Build history of the part. All positions in model axes, mm. Give positions to 0.01 mm unless a question says otherwise; leave off trailing zeros. Write each loop counter-clockwise with the first axis right and the second up, starting at its lowest first coordinate (ties: lowest second). Pieces come first, ordered by that corner, then holes. Notation, with made-up numbers: (0, 71.25) -> (43, 71.25) arc R18 cw to (43, 91.25) -> close; hole circle Ø8 at (-17.5, -27). An arc over 180 degrees is marked (long way). Put each result on its own line as item: value. Start each with the question number.
Item 1: Drill centre lines: line 1 along Y through (x, z) = (0.5, -5); line 2 along X through (y, z) = (18.5, -2.25); line 3 along Y through (x, z) = (0, -1.5). Where is each one in solid material? Low to high.
Item 2: Two-plate mould, pull along Y, no slides. Class faces 1 (the cylindrical face through (5.961, -26.846, -0.14)), 2 (the flat face through (-17, -22, -10)): pulls with the +Y half, pulls with the -Y half, needs draft (parallel to the pull), parting line crosses it, or undercut.
Item 3: Slice it at C-C, the plane z = -3. List the corners of the cut face in (x, y), plus the area to 3 significant figures.
Item 4: Slice it at A-A, the plane y = 0. List the corners of the cut face in (x, z), plus the area to 3 significant figures.
Item 5: Flat gauge pins, fed straight in: pin 1 Ø8 at (x, z) = (21.5, 4.5) entering from -Y; pin 2 Ø1.5 at (x, z) = (18, -8) entering from -Y; pin 3 Ø5 at (x, z) = (27, 3) entering from -Y; pin 4 Ø12 at (x, y) = (24, -24.5) entering from -Z. Where does each tip first touch, or does it go through?
```python
from build123d import *

# Parameters (mm, degrees)
SKETCH_2_R               = 5
EXTRUDE_1_DEPTH          = 10
PATTERN_CIRCULAR_1_COUNT = 6
EXTRUDE_2_DEPTH          = 7
SKETCH_4_R               = 1.4
CUT_EXTRUDE_1_DEPTH      = 50.325449958
PATTERN_CIRCULAR_2_COUNT = 6
SKETCH_5_R               = 5.5
EXTRUDE_3_DEPTH          = 5
SKETCH_7_R               = 7
CUT_EXTRUDE_3_DEPTH      = 1.5
CUT_EXTRUDE_3_DRAFT      = -40
SKETCH_8_R               = 1.5
CUT_EXTRUDE_4_DEPTH      = 51.222007264
SKETCH_10_R              = 1.25
CUT_EXTRUDE_6_DEPTH      = 51.675437971
PATTERN_CIRCULAR_3_COUNT = 6
SKETCH_11_R              = 2.5
CUT_EXTRUDE_7_DEPTH      = 51.675437971
PATTERN_CIRCULAR_4_COUNT = 2
CUT_EXTRUDE_8_DEPTH      = 8
PATTERN_CIRCULAR_5_COUNT = 6
CUT_EXTRUDE_9_DEPTH      = 8
SKETCH_14_R              = 27.5
CUT_EXTRUDE_11_DEPTH     = 55


with BuildPart() as part:
    # 草图1 → 旋转1 (revolve)
    with BuildSketch(Plane(origin=(0, 0, 0), x_dir=(1, 0, 0), z_dir=(0, 1, 0)), mode=Mode.PRIVATE) as revolve_1_sk:
        with BuildLine():
            Line((25, 10), (25, -10))
            Line((25, -10), (29, -10))
            ThreePointArc((29, -10), (33.787135539, -6.443375673), (31.763853992, -0.833333333))
            ThreePointArc((31.763853992, -0.833333333), (31.31662479, 0), (31.763853992, 0.833333333))
            ThreePointArc((31.763853992, 0.833333333), (33.787135539, 6.443375673), (29, 10))
            Line((29, 10), (25, 10))
        make_face()
    revolve(revolve_1_sk.sketch.rotate(Axis((0, 0, -146.934042126), (0, 0, 1)), 180), axis=Axis((0, 0, -146.934042126), (0, 0, 1)))

    # 草图2 → 凸台-拉伸1 (add)
    with BuildSketch(Plane.XY.offset(6)):
        with Locations((0, 21.5)):
            Circle(SKETCH_2_R)
    extrude_1 = extrude(amount=-EXTRUDE_1_DEPTH)

    # 阵列(圆周)1: 凸台-拉伸1 ×6 about axis
    pattern_circular_1_axis = Axis((0, 0, 0), (0, 0, 1))
    for i in range(1, PATTERN_CIRCULAR_1_COUNT):
        add(extrude_1.rotate(pattern_circular_1_axis, i * 360 / PATTERN_CIRCULAR_1_COUNT))

    # 草图3 → 凸台-拉伸2 (add)
    with BuildSketch(Plane.XY.offset(6)):
        with BuildLine():
            Line((-8.082903769, 0), (-10.874355653, -4.834936491))
            Line((-10.874355653, -4.834936491), (-15.051918724, -7.246853654))
            ThreePointArc((-15.051918724, -7.246853654), (-14.289419162, -8.25), (-13.801918724, -9.411917163))
            Line((-13.801918724, -9.411917163), (-9.624355653, -7))
            Line((-9.624355653, -7), (-4.041451884, -7))
            Line((-4.041451884, -7), (-1.25, -11.834936491))
            Line((-1.25, -11.834936491), (-1.25, -16.658770817))
            ThreePointArc((-1.25, -16.658770817), (0, -16.5), (1.25, -16.658770817))
            Line((1.25, -16.658770817), (1.25, -11.834936491))
            Line((1.25, -11.834936491), (4.041451884, -7))
            Line((4.041451884, -7), (9.624355653, -7))
            Line((9.624355653, -7), (13.801918724, -9.411917163))
            ThreePointArc((13.801918724, -9.411917163), (14.289419162, -8.25), (15.051918724, -7.246853654))
            Line((15.051918724, -7.246853654), (10.874355653, -4.834936491))
            Line((10.874355653, -4.834936491), (8.082903769, 0))
            Line((8.082903769, 0), (10.874355653, 4.834936491))
            Line((10.874355653, 4.834936491), (15.051918724, 7.246853654))
            ThreePointArc((15.051918724, 7.246853654), (14.289419162, 8.25), (13.801918724, 9.411917163))
            Line((13.801918724, 9.411917163), (9.624355653, 7))
            Line((9.624355653, 7), (4.041451884, 7))
            Line((4.041451884, 7), (1.25, 11.834936491))
            Line((1.25, 11.834936491), (1.25, 16.658770817))
            ThreePointArc((1.25, 16.658770817), (0, 16.5), (-1.25, 16.658770817))
            Line((-1.25, 16.658770817), (-1.25, 11.834936491))
            Line((-1.25, 11.834936491), (-4.041451884, 7))
            Line((-4.041451884, 7), (-9.624355653, 7))
            Line((-9.624355653, 7), (-13.801918724, 9.411917163))
            ThreePointArc((-13.801918724, 9.411917163), (-14.289419162, 8.25), (-15.051918724, 7.246853654))
            Line((-15.051918724, 7.246853654), (-10.874355653, 4.834936491))
            Line((-10.874355653, 4.834936491), (-8.082903769, 0))
        make_face()
    extrude(amount=-EXTRUDE_2_DEPTH)

    # 草图4 → 切除-拉伸1 (cut, through all)
    with BuildSketch(Plane(origin=(0, 0, -1), x_dir=(-1, 0, 0), z_dir=(0, 0, -1))):
        with Locations((0, 8.5)):
            Circle(SKETCH_4_R)
    cut_extrude_1 = extrude(amount=-CUT_EXTRUDE_1_DEPTH, mode=Mode.SUBTRACT)

    # 阵列(圆周)2: 切除-拉伸1 ×6 about axis
    pattern_circular_2_axis = Axis((0, 0, 0), (0, 0, 1))
    for i in range(1, PATTERN_CIRCULAR_2_COUNT):
        add(cut_extrude_1.rotate(pattern_circular_2_axis, i * 360 / PATTERN_CIRCULAR_2_COUNT), mode=Mode.SUBTRACT)

    # 草图5 → 凸台-拉伸3 (add)
    with BuildSketch(Plane(origin=(0, 0, -1), x_dir=(-1, 0, 0), z_dir=(0, 0, -1))):
        with Locations(Location((0, 0, 0), (0, 0, 180))):
            Circle(SKETCH_5_R)
    extrude(amount=EXTRUDE_3_DEPTH)


with BuildPart() as cut_extrude_3_tool:
    # 草图7 → 切除-拉伸3 (with draft: the straight prism first)
    with BuildSketch(Plane.XY.offset(6)):
        Circle(SKETCH_7_R)
    extrude(amount=-CUT_EXTRUDE_3_DEPTH)
    # 切除-拉伸3: the draft: its side faces are tilted about the plane it starts from
    cut_extrude_3_sides = [cut_extrude_3_tool.faces().sort_by_distance(p)[0] for p in [
        (-7, 0, 5.25),
    ]]
    draft(cut_extrude_3_sides, Plane.XY.offset(6), CUT_EXTRUDE_3_DRAFT)


with BuildPart() as part_1:
    add(part.part)

    # 切除-拉伸3: cut by cut_extrude_3_tool
    add(cut_extrude_3_tool.part, mode=Mode.SUBTRACT)

    # 草图8 → 切除-拉伸4 (cut, through all)
    with BuildSketch(Plane.XY.offset(4.5)):
        Circle(SKETCH_8_R)
    extrude(amount=-CUT_EXTRUDE_4_DEPTH, mode=Mode.SUBTRACT)

    # 草图10 → 切除-拉伸6 (cut, through all)
    with BuildSketch(Plane.XY.offset(6)):
        with Locations((0, 21.5)):
            Circle(SKETCH_10_R)
    cut_extrude_6 = extrude(amount=-CUT_EXTRUDE_6_DEPTH, mode=Mode.SUBTRACT)

    # 阵列(圆周)3: 切除-拉伸6 ×6 about axis
    pattern_circular_3_axis = Axis((0, 0, 0), (0, 0, 1))
    for i in range(1, PATTERN_CIRCULAR_3_COUNT):
        add(cut_extrude_6.rotate(pattern_circular_3_axis, i * 360 / PATTERN_CIRCULAR_3_COUNT), mode=Mode.SUBTRACT)

    # 草图11 → 切除-拉伸7 (cut, through all)
    with BuildSketch(Plane.XY.offset(6)):
        with Locations((0, 21.5)):
            Circle(SKETCH_11_R)
    cut_extrude_7 = extrude(amount=-CUT_EXTRUDE_7_DEPTH, mode=Mode.SUBTRACT)

    # 阵列(圆周)4: 切除-拉伸7 ×2 about axis
    pattern_circular_4_axis = Axis((0, 0, 0), (0, 0, 1))
    for i in range(1, PATTERN_CIRCULAR_4_COUNT):
        add(cut_extrude_7.rotate(pattern_circular_4_axis, i * 360 / PATTERN_CIRCULAR_4_COUNT), mode=Mode.SUBTRACT)

    # 草图12 → 切除-拉伸8 (cut)
    with BuildSketch(Plane.XY.offset(6)):
        Polygon((20.062921854, 8.25), (21.506297527, 10.75), (20.062921854, 13.25), (17.176170508, 13.25), (15.732794835, 10.75), (17.176170508, 8.25), align=None)
    cut_extrude_8 = extrude(amount=-CUT_EXTRUDE_8_DEPTH, mode=Mode.SUBTRACT)

    # 阵列(圆周)5: 切除-拉伸8 ×6 about axis, 2 skipped
    pattern_circular_5_axis = Axis((0, 0, 0), (0, 0, -1))
    add([cut_extrude_8.rotate(pattern_circular_5_axis, i * 360 / PATTERN_CIRCULAR_5_COUNT) for i in range(1, PATTERN_CIRCULAR_5_COUNT) if i not in (2, 5)], mode=Mode.SUBTRACT)

    # 草图9 → 切除-拉伸9 (cut)
    with BuildSketch(Plane(origin=(0, 0, -6), x_dir=(-1, 0, 0), z_dir=(0, 0, -1))):
        Polygon((3.5, 0), (1.75, 3.031088913), (-1.75, 3.031088913), (-3.5, 0), (-1.75, -3.031088913), (1.75, -3.031088913), align=None)
    extrude(amount=-CUT_EXTRUDE_9_DEPTH, mode=Mode.SUBTRACT)

    # 草图14 → 切除-拉伸11 (cut)
    with BuildSketch(Plane(origin=(0, 0, -10), x_dir=(-1, 0, 0), z_dir=(0, 0, -1))):
        Circle(SKETCH_14_R)
    extrude(amount=-CUT_EXTRUDE_11_DEPTH, mode=Mode.SUBTRACT)


solid = part_1.part
```
Values follow:
1. line 1: -34 to -27.5, 27.5 to 34
1. line 2: -27.54 to -20.35, 20.35 to 27.54
1. line 3: -32.57 to -27.5, 27.5 to 32.57
2. face 1: undercut
2. face 2: needs draft
3. outline: circle Ø67.17 at (0, 0); hole circle Ø55 at (0, 0)
3. area: 1,170 mm2
4. outline: (-31.76, -0.83) arc R5 ccw to (-29, -10) -> (-27.5, -10) -> (-27.5, 10) -> (-29, 10) arc R5 ccw to (-31.76, 0.83) arc R1 cw to start; (27.5, -10) -> (29, -10) arc R5 ccw to (31.76, -0.83) arc R1 cw to (31.76, 0.83) arc R5 ccw to (29, 10) -> (27.5, 10) -> close
4. area: 219 mm2
5. pin 1: y = -29.14
5. pin 2: y = -28.41
5. pin 3: y = -23.22
5. pin 4: z = -10
